Could you check a few things on this model? Use its own coordinates, in mm. Face numbers are marked on the shaded views. A direction names the side the tool comes from. Round coordinates to 2 decimals unless told otherwise and drop trailing zeros. Loops run counter-clockwise (first coordinate to the right, second up) from the corner with the lowest first, then second, coordinate; pieces in that order, holes last. Notation, with made-up numbers: M -30,3 L -12,3 A16 ccw -12,7 Z; hole C -12.75,65.5 d9. An arc over 180 degrees is marked long. Answer in a Markdown table with one row per item.
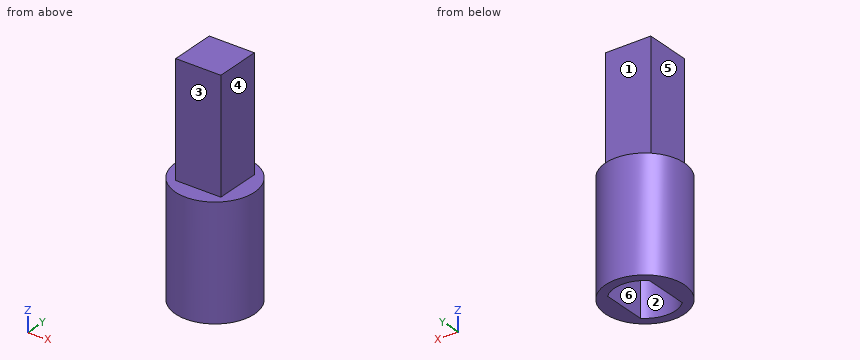
Autodesk Inventor part; units mm, degrees
ref_plane "YZ Plane" through (0, 0, 0) normal (1, 0, 0) x (0, 1, 0)
ref_plane "XZ Plane" through (0, 0, 0) normal (0, 1, 0) x (-1, 0, 0)
ref_plane "XY Plane" through (0, 0, 0) normal (0, 0, 1) x (1, 0, 0)
sketch "Sketch1" plane through (0, 0, 0) normal (0, 0, 1) x (1, 0, 0)
  circle A0 centre (0, 0) radius 3.5
  line L0 (1.86, 1.9571) -> (1.86, -1.9571)
  line L1 (0, 3.5) -> (0, -3.5)
  line L2 (-1.86, 1.9571) -> (-1.86, -1.9571)
  arc A1 (-1.86, -1.9571) -> (1.86, -1.9571) centre (0, 0) ccw
  arc A2 (1.86, 1.9571) -> (-1.86, 1.9571) centre (0, 0) ccw
  dimension "d0" = 7
  dimension "d1" = 2.7
  dimension "d2" = 3.72
extrude "Extrusion1" add sketch "Sketch1" along normal blind 7 contours A0 L1 A1 L0 A2 | L1 A2 L2 A1 A0
sketch "Sketch2" plane through (0, 0, 7) normal (0, 0, 1) x (1, 0, 0)
  circle A0 centre (0, 0) radius 3.5
  circle A1 centre (0, 0) radius 3.5
extrude "Extrusion2" add sketch "Sketch2" along normal blind 3
sketch "Sketch3" plane through (0, 0, 10) normal (0, 0, 1) x (1, 0, 0)
  line L0 (-2, -2) -> (2, -2)
  line L1 (2, -2) -> (2, 2)
  line L2 (2, 2) -> (-2, 2)
  line L3 (-2, 2) -> (-2, -2)
  line L4 (-2, -2) -> (2, 2) construction
  line L5 (2, -2) -> (-2, 2) construction
  point P0 (0, 0)
  dimension "d7" = 4
  dimension "d8" = 4
extrude "Extrusion3" add sketch "Sketch3" along normal blind 10
properties part number "Geared Motor Transmission"
1) Which directions (+Z, -Z, +X, -X, +Y, -Y) give clear straight access to the entire face, cutting with the end or side of a thin tool? Please do the marked faces 4, 5 and 6.
Computed:
| item | result |
|---|---|
| face 4 | +Z, +X, +Y, -Y |
| face 5 | +Z, -X, +Y, -Y |
| face 6 | -Z |
2) I want a section at D-D, the plane z = 16.25. Please give me the cut outline in (x, y).
Computed:
| item | result |
|---|---|
| outline | M -2,-2 L 2,-2 L 2,2 L -2,2 Z |
3) If we mould it in two halves opening along Y, with no side actions, what happens to the marked faces 1, 2 and 3? For each: released by +Y, released by -Y, zero draft, split by the parting line, or undercut.
Computed:
| item | result |
|---|---|
| face 1 | released by +Y |
| face 2 | undercut |
| face 3 | released by -Y |
4) I need wall thicknesses on line 1 (Z direction, x = -1, y = -1.5); line 2 (X direction, y = 0.75, z = 12.5); line 3 (X direction, y = 1.25, z = 5.5). Which ranges of each line are inside material? Lowest first, please.
Computed:
| item | result |
|---|---|
| line 1 | z = 7 to 20 |
| line 2 | x = -2 to 2 |
| line 3 | x = -3.27 to -1.86, 1.86 to 3.27 |
5) I want a section at A-A, the plane x = 0. Please give me the cut outline in (y, z), plus the area to 3 significant figures.
Computed:
| item | result |
|---|---|
| outline | M -3.5,0 L -2.7,0 L -2.7,7 L 2.7,7 L 2.7,0 L 3.5,0 L 3.5,10 L 2,10 L 2,20 L -2,20 L -2,10 L -3.5,10 Z |
| area | 72.2 mm² |
6) I want a section at B-B, the plane z = 6. Please give me the cut outline in (x, y), plus the area to 3 significant figures.
Computed:
| item | result |
|---|---|
| outline | C 0,0 d7; hole M -1.86,-1.96 A2.7 ccw 1.86,-1.96 L 1.86,1.96 A2.7 ccw -1.86,1.96 Z |
| area | 20.1 mm² |
7) I want a section at C-C, the plane y = -0.25. Please give me the cut outline in (x, z).
Computed:
| item | result |
|---|---|
| outline | M -3.49,0 L -1.86,0 L -1.86,7 L 1.86,7 L 1.86,0 L 3.49,0 L 3.49,10 L 2,10 L 2,20 L -2,20 L -2,10 L -3.49,10 Z |
8) Will these pins go through, and if not, where does the flat tip stop? P1, Ø1.2, axis at y = -0.5, z = 16, coming from the +X side; P2, Ø1.1, axis at x = 1, y = 0, coming from the -Z side; P3, Ø3, axis at x = 1, z = 12.5, coming from the +Y side.
Computed:
| item | result |
|---|---|
| P1 | stops at x = 2 |
| P2 | stops at z = 7 |
| P3 | stops at y = 2 |
